Here's how the part is built. I have some questions about the finished solid (model axes, mm). A direction names the side the tool comes from. Round coordinates to 2 decimals unless told otherwise and drop trailing zeros. Write each loop counter-clockwise with the first axis right and the second up, starting at its lowest first coordinate (ties: lowest second). Pieces come first, ordered by that corner, then holes. Notation, with made-up numbers: (23, 17.25) -> (72, 17.25) arc R31 ccw to (72, 44.25) -> close; hole circle Ø1 at (81, 20.5). An arc over 180 degrees is marked (long way). Answer in a Markdown table with one row per item.
from build123d import *

# Parameters (mm, degrees)
F1_DEPTH  = 5
F3_DEPTH  = 25
F4_W      = 5
F4_H      = 5
F5_DEPTH  = 25
F6_W      = 5
F6_H      = 5
F7_DEPTH  = 25
F8_W      = 4.95
F8_H      = 4.95
F9_DEPTH  = 25
F10_W     = 4.95
F10_H     = 4.95
F11_DEPTH = 25


with BuildPart() as f1:
    # F0 (on Top) → F1 (new body)
    with BuildSketch(Plane.XY):
        Polygon((5, 25), (0, 25), (0, -25), (5, -25), (5, -45), (10, -45), (10, -40), (15, -40), (15, -30), (25, -30), (25, -45), (30, -45), (30, -40), (35, -40), (35, -30), (55, -30), (55, -45), (60, -45), (60, -40), (65, -40), (65, -30), (75, -30), (75, -45), (80, -45), (80, -40), (85, -40), (85, -20), (90, -20), (90, 25), (85, 25), (85, 10), (70, 10), (70, 15), (60, 15), (60, 20), (50, 20), (50, 30), (45, 30), (45, 40), (40, 40), (40, 35), (35, 35), (35, 40), (15, 40), (15, 35), (10, 35), (10, 40), (5, 40), align=None)
    extrude(amount=F1_DEPTH)

    # F2 (on face) → F3 (cut)
    with BuildSketch(Plane.XY.offset(5)):
        Polygon((15, 5), (10, 5), (10, 0), (30, 0), (30, 5), (20, 5), (20, 10), (25, 10), (25, 15), (15, 15), align=None)
    extrude(amount=-F3_DEPTH, mode=Mode.SUBTRACT)

    # F4 (on face) → F5 (cut)
    with BuildSketch(Plane.XY.offset(5)):
        with Locations((12.5, 22.5)):
            Rectangle(F4_W, F4_H)
    extrude(amount=-F5_DEPTH, mode=Mode.SUBTRACT)

    # F6 (on face) → F7 (cut)
    with BuildSketch(Plane.XY.offset(5)):
        with Locations((27.5, 22.5)):
            Rectangle(F6_W, F6_H)
    extrude(amount=-F7_DEPTH, mode=Mode.SUBTRACT)

    # F8 (on face) → F9 (cut)
    with BuildSketch(Plane.XY.offset(5)):
        with Locations((7.475, 7.475)):
            Rectangle(F8_W, F8_H)
    extrude(amount=-F9_DEPTH, mode=Mode.SUBTRACT)

    # F10 (on face) → F11 (cut)
    with BuildSketch(Plane.XY.offset(5)):
        with Locations((32.495, 7.525)):
            Rectangle(F10_W, F10_H)
    extrude(amount=-F11_DEPTH, mode=Mode.SUBTRACT)


solid = f1.part
1) I need wall thicknesses on line 1 (Y direction, x = 13, z = 1.3); line 2 (X direction, y = 21, z = 3.2); line 3 (X direction, y = 14, z = 3.2). Which ranges of each line are inside material? Lowest first, please. Write a range as [from, to].
Response:
| item | result |
|---|---|
| line 1 | y = [-40, 0], [5, 20], [25, 35] |
| line 2 | x = [0, 10], [15, 25], [30, 50], [85, 90] |
| line 3 | x = [0, 15], [25, 70], [85, 90] |
2) Which directions (+Z, -Z, +X, -X, +Y, -Y) give clear straight access to the entire face, cutting with the end or side of a thin tool? Please do faces 5 (the face through (32, -40, 2)), 6 (the face through (3, 25, 2)), 7 (the face through (87, -20, 2)), 8 (the face through (20, 15, 3)), 9 (the face through (85, 18, 2)).
Response:
| item | result |
|---|---|
| face 5 | +Z, -Z, -Y |
| face 6 | +Z, -Z, -X, +Y |
| face 7 | +Z, -Z, +X, -Y |
| face 8 | +Z, -Z |
| face 9 | +Z, -Z, +Y |
3) For pin 1 (1.5 mm diameter, centred on x = 44, z = 2.5, fed in from -Y); pin 2 (1.5 mm diameter, centred on y = 34, z = 2, fed in from -X); pin 3 (2.5 mm diameter, centred on x = 66, z = 1.5, fed in from +Y), each with a flat end and sliding along its axis, tell me the tip position at first contact or that it passes through.
Response:
| item | result |
|---|---|
| pin 1 | stops at y = -30 |
| pin 2 | stops at x = 5 |
| pin 3 | stops at y = 15 |
4) We'd pull the mould along X, two halves only. Please class faces 1 (the face through (15, 22, 3)), 2 (the face through (77, -45, 2)), 3 (the face through (30, 22, 3)), 4 (the face through (45, 35, 2)): +X half, -X half, draft (parallel to the pull), parting line (faces both ways), or undercut.
Response:
| item | result |
|---|---|
| face 1 | undercut |
| face 2 | draft |
| face 3 | undercut |
| face 4 | +X half |
5) I want a section at A-A, the plane y = -36.5. List the corners of the cut face in (x, z) for me, and give its area (3 significant figures).
Response:
| item | result |
|---|---|
| outline | (5, 0) -> (15, 0) -> (15, 5) -> (5, 5) -> close; (25, 0) -> (35, 0) -> (35, 5) -> (25, 5) -> close; (55, 0) -> (65, 0) -> (65, 5) -> (55, 5) -> close; (75, 0) -> (85, 0) -> (85, 5) -> (75, 5) -> close |
| area | 200 mm^2 |
6) I want a section at C-C, the plane y = 12.5. List the corners of the cut face in (x, z) for me, and give its area (3 significant figures).
Response:
| item | result |
|---|---|
| outline | (0, 0) -> (15, 0) -> (15, 5) -> (0, 5) -> close; (25, 0) -> (70, 0) -> (70, 5) -> (25, 5) -> close; (85, 0) -> (90, 0) -> (90, 5) -> (85, 5) -> close |
| area | 325 mm^2 |
7) I want a section at D-D, the plane z = 3.9. Count the separate pieces of the cut face and the enclosed holes in it, and give its area (3 significant figures).
Response:
| item | result |
|---|---|
| separate pieces | 1 |
| enclosed holes | 5 |
| area | 5,300 mm^2 |
8) I want a section at B-B, the plane x = 28. List the corners of the cut face in (y, z) for me, and give its area (3 significant figures).
Response:
| item | result |
|---|---|
| outline | (-45, 0) -> (0, 0) -> (0, 5) -> (-45, 5) -> close; (5, 0) -> (20, 0) -> (20, 5) -> (5, 5) -> close; (25, 0) -> (40, 0) -> (40, 5) -> (25, 5) -> close |
| area | 375 mm^2 |
